Drawing for the job (mm, zero at the part's lowest x, y, z). A direction names the side the tool comes from. Coordinates: 2 decimals unless noted, no trailing zeros. Order: outer loops, then holes, each group sorted by start corner. A loop starts at its lowest first (then second) coordinate and runs counter-clockwise, first axis right, second up.
1) Cut at A-A (y = 20.5). List the corners of the cut face in (x, z).
2) Cut at D-D (y = 29). List the corners of the cut face in (x, z), and give its area (3 significant figures).
3) Wall check: L1, parallel to Y at x = 19, z = 70; L2, parallel to X at y = 30.5, z = 55; L3, parallel to Y at x = 12.5, z = 47.5. Give the ranges that are in metal, low to high.
4) Mould opens along Z. For the marked faces 5, 6, 7 and 8 say: +Z half, -Z half, draft (parallel to the pull), parting line (faces both ways), or undercut.
5) Pin check, flat tips, straight feed: pin 1 Ø8 at (y, z) = (15, 51.5) entering from +X; pin 2 Ø6.5 at (x, z) = (8, 48.5) entering from -Y; pin 3 Ø12 at (x, z) = (32, 66) entering from -Y. Stop position of each tip, or through.
6) Cut at C-C (z = 47.5). List the corners of the cut face in (x, y), and give its area (3 significant figures).
7) Cut at B-B (x = 6.5). List the corners of the cut face in (y, z), and give its area (3 significant figures).
8) Tool access for the marked faces 1, 2, 3 and 4: list every direction of +Z, -Z, +X, -X, +Y, -Y with a clear straight run to the whole face (end or side of a thin tool).
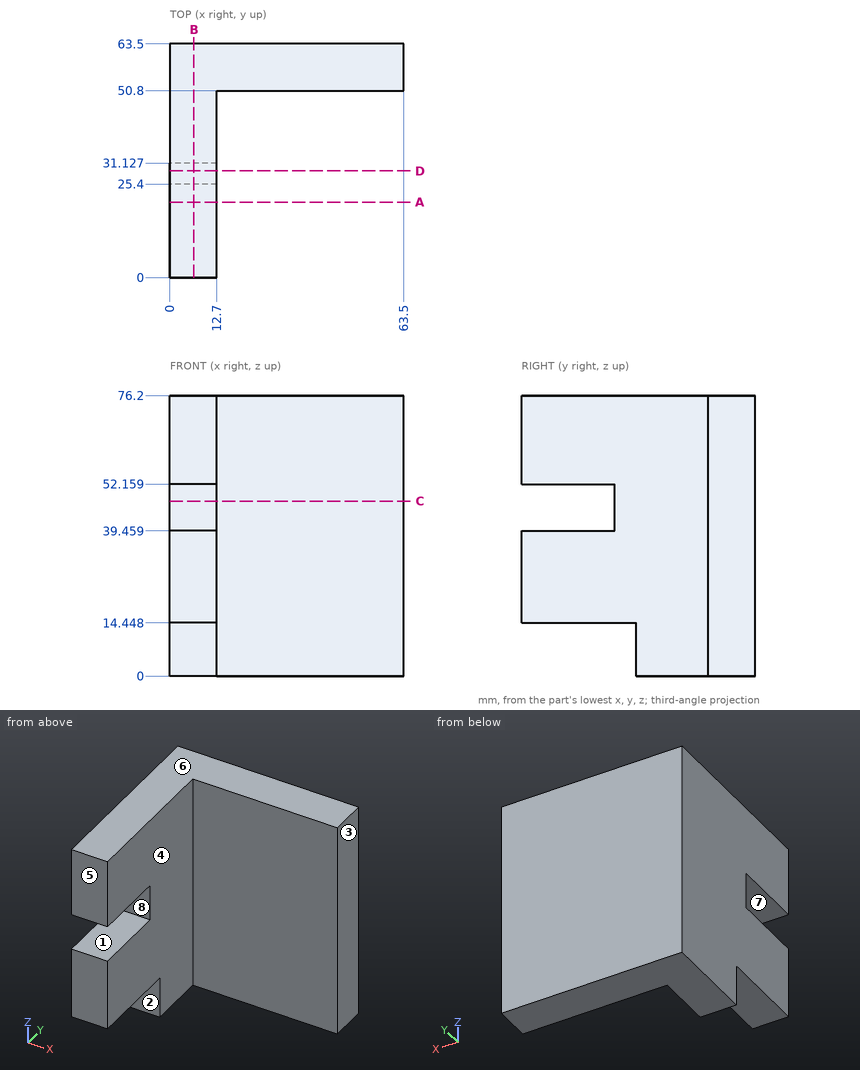
Geometry check:
1. outline: (0, 14.45) - (12.7, 14.45) - (12.7, 39.46) - (0, 39.46) - close; (0, 52.16) - (12.7, 52.16) - (12.7, 76.2) - (0, 76.2) - close
2. outline: (0, 14.45) - (12.7, 14.45) - (12.7, 76.2) - (0, 76.2) - close
2. area: 784 mm2
3. L1: y = 50.8 to 63.5
3. L2: x = 0 to 12.7
3. L3: y = 25.4 to 63.5
4. face 5: draft
4. face 6: +Z half
4. face 7: undercut
4. face 8: undercut
5. pin 1: stops at x = 12.7
5. pin 2: stops at y = 25.4
5. pin 3: stops at y = 50.8
6. outline: (0, 25.4) - (12.7, 25.4) - (12.7, 50.8) - (63.5, 50.8) - (63.5, 63.5) - (0, 63.5) - close
6. area: 1,130 mm2
7. outline: (0, 14.45) - (31.13, 14.45) - (31.13, 0) - (63.5, 0) - (63.5, 76.2) - (0, 76.2) - (0, 52.16) - (25.4, 52.16) - (25.4, 39.46) - (0, 39.46) - close
7. area: 4,070 mm2
8. face 1: +X, -X, -Y
8. face 2: -Z, +X, -X, -Y
8. face 3: +Z, -Z, +X, +Y, -Y
8. face 4: +Z, -Z, +X, -Y
